Autodesk Inventor part; units mm, degrees
ref_plane "YZ Plane" through (0, 0, 0) normal (1, 0, 0) x (0, 1, 0)
ref_plane "XZ Plane" through (0, 0, 0) normal (0, 1, 0) x (-1, 0, 0)
ref_plane "XY Plane" through (0, 0, 0) normal (0, 0, 1) x (1, 0, 0)
sketch "Sketch1" plane through (0, 0, 0) normal (0, 1, 0) x (-1, 0, 0)
  circle A0 centre (0, 0) radius 2.159
  circle A1 centre (0, 38.1) radius 2.159
  circle A2 centre (0, 38.1) radius 4.5403
  circle A3 centre (0, 0) radius 4.5403
  line L0 (4.5403, 38.1) -> (4.5402, 0)
  line L1 (-4.5403, 0) -> (-4.5403, 38.1)
  dimension "d0" = 4.318
  dimension "d1" = 4.318
  dimension "d2" = 38.1
  dimension "d3" = 2.3813
  dimension "d4" = 2.3813
extrude "Extrusion1" add sketch "Sketch1" along normal blind 3.175
properties part number "Arm for thingy"
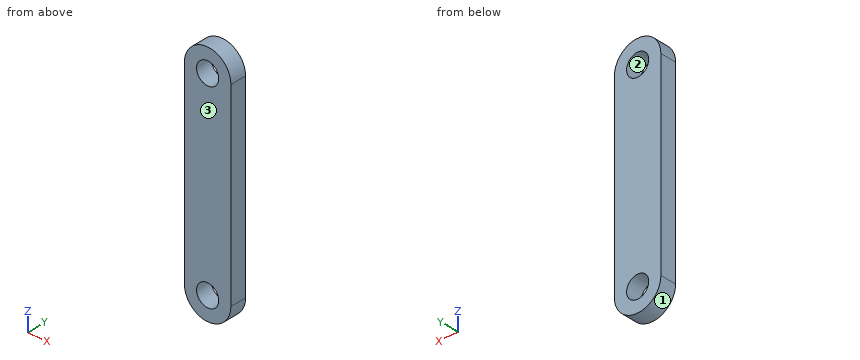
Model file for the job. Use its own axes, mm. Face numbers are marked on the shaded views. Round coordinates to 2 decimals unless told otherwise and drop trailing zeros. Write each loop counter-clockwise with the first axis right and the second up, starting at its lowest first coordinate (ties: lowest second). Pieces come first, ordered by that corner, then holes. Notation, with made-up numbers: (59.5, 76) - (66.5, 76) arc R34 cw to (66.5, 114) - close; hole circle Ø3 at (58.5, 51). An arc over 180 degrees is marked (long way). One line per item, written item: value.
(1) Two-plate mould, pull along X, no slides. Class the marked faces 1, 2 and 3: pulls with the +X half, pulls with the -X half, needs draft (parallel to the pull), parting line crosses it, or undercut.
Values follow:
face 1: parting line crosses it
face 2: undercut
face 3: needs draft
(2) Cut at B-B, the plane y = 2. Give the cut face in (x, z), plus the area to 3 significant figures.
Values follow:
outline: (-4.54, 0) arc R4.54 ccw to (4.54, 0) - (4.54, 38.1) arc R4.54 ccw to (-4.54, 38.1) - close; hole circle Ø4.32 at (0, 0); hole circle Ø4.32 at (0, 38.1)
area: 381 mm²
(3) Drop a flat-ended pin along its axis: P1, Ø5, axis at x = 3.5, z = 16.5, coming from the -Y side. Give the stop position or say it passes through.
Values follow:
P1: stops at y = 0
(4) Cut at C-C, the plane x = -1.75. Give the cut face in (y, z) (3 decimals).
Values follow:
outline: (0, -4.189) - (3.175, -4.189) - (3.175, -1.264) - (0, -1.264) - close; (0, 1.264) - (3.175, 1.264) - (3.175, 36.836) - (0, 36.836) - close; (0, 39.364) - (3.175, 39.364) - (3.175, 42.289) - (0, 42.289) - close
(5) Wall check: probe 1 along Z at (x, y) = (0, 0.85); probe 2 along Z at (x, y) = (1.5, 0.3); probe 3 along Z at (x, y) = (-3, 0.3). Give the ranges that are in metal, low to high.
Values follow:
probe 1: z = -4.54 to -2.16, 2.16 to 35.94, 40.26 to 42.64
probe 2: z = -4.29 to -1.55, 1.55 to 36.55, 39.65 to 42.39
probe 3: z = -3.41 to 41.51
(6) Cut at A-A, the plane x = 0. Give the cut face in (y, z) (3 decimals), plus the area to 3 significant figures.
Values follow:
outline: (0, -4.54) - (3.175, -4.54) - (3.175, -2.159) - (0, -2.159) - close; (0, 2.159) - (3.175, 2.159) - (3.175, 35.941) - (0, 35.941) - close; (0, 40.259) - (3.175, 40.259) - (3.175, 42.64) - (0, 42.64) - close
area: 122 mm²
(7) Cut at D-D, the plane x = -4. Give the cut face in (y, z) (3 decimals), plus the area to 3 significant figures.
Values follow:
outline: (0, -2.148) - (3.175, -2.148) - (3.175, 40.248) - (0, 40.248) - close
area: 135 mm²
